from build123d import *

# Parameters (mm, degrees)
ESQUISSE1_R         = 20
ESQUISSE1_R_2       = 12.7
BOSS_EXTRU_1_DEPTH  = 8.78
ESQUISSE2_R         = 38
ESQUISSE2_R_2       = 11.2
BOSS_EXTRU_2_DEPTH  = 47.8
CHANFREIN3_SIZE     = 11.200084029
CHANFREIN3_SIZE_2   = 49.8
SKETCH7_R           = 38
SKETCH7_R_2         = 26
CUT_EXTRUDE2_DEPTH  = 3
CIRPATTERN1_COUNT   = 3
CIRPATTERN2_COUNT   = 3
SKETCH23_R          = 13.7
SKETCH23_R_2        = 12.6
BOSS_EXTRUDE1_DEPTH = 0.3
LPATTERN1_COUNT     = 8
LPATTERN1_PITCH     = 5


with BuildPart() as part:
    # Esquisse1 → Boss.-Extru.1 (new body)
    with BuildSketch(Plane.XY):
        Circle(ESQUISSE1_R)
        Circle(ESQUISSE1_R_2, mode=Mode.SUBTRACT)
    extrude(amount=BOSS_EXTRU_1_DEPTH)

    # Esquisse2 → Boss.-Extru.2 (add)
    with BuildSketch(Plane(origin=(0, 0, 0), x_dir=(-1, 0, 0), z_dir=(0, 0, -1))):
        with Locations(Location((0, 0, 0), (0, 0, 180))):
            Circle(ESQUISSE2_R)
        with Locations(Location((0, 0, 0), (0, 0, 180))):
            Circle(ESQUISSE2_R_2, mode=Mode.SUBTRACT)
    extrude(amount=BOSS_EXTRU_2_DEPTH)

    # Chanfrein3
    # the kernel refuses this chamfer: 49.8, 11.200084029 mm, written as the material it takes off along each edge
    with BuildSketch(Plane(origin=(0, 0, -47.8), x_dir=(1, 0, 0), z_dir=(0, 1, 0))) as chanfrein3_piece_1:
        Polygon((11.2 + CHANFREIN3_SIZE, 0), (11.2, -CHANFREIN3_SIZE_2), (11.2, 0), align=None)
    revolve(axis=Axis((0, 0, -47.8), (0, 0, -1)), mode=Mode.SUBTRACT)

    # Sketch7 → Cut-Extrude2 (cut)
    with BuildSketch(Plane.XY):
        Circle(SKETCH7_R)
        Circle(SKETCH7_R_2, mode=Mode.SUBTRACT)
    cut_extrude2 = extrude(amount=-CUT_EXTRUDE2_DEPTH, mode=Mode.SUBTRACT)

    # Sketch19 → Hole for #4 300® SC Nuts (SP)2 (revolve, cut)
    with BuildSketch(Plane(origin=(28.837585054, 8.270047658, -47.8), x_dir=(0, 1, 0), z_dir=(1, 0, 0))):
        Polygon((0, 0), (0, 6.266734357), (2.1082, 5), (2.1082, 0), align=None)
    hole_for_4_300_sc_nuts_sp_2 = revolve(axis=Axis((28.837585054, 8.270047658, -54.15), (0, 0, 1)), mode=Mode.SUBTRACT)

    # CirPattern1: Hole for #4 300® SC Nuts (SP)2 ×3 about axis
    cirpattern1_axis = Axis((0, 0, 0), (0, 0, 1))
    for i in range(1, CIRPATTERN1_COUNT):
        add(hole_for_4_300_sc_nuts_sp_2.rotate(cirpattern1_axis, i * 360 / CIRPATTERN1_COUNT), mode=Mode.SUBTRACT)

    # Sketch22 → Hole for #4 300® SC Nuts (SP)3 (revolve, cut)
    with BuildSketch(Plane(origin=(15.86067178, 4.548526212, 8.78), x_dir=(0, -1, 0), z_dir=(1, 0, 0))):
        Polygon((0, 0), (0, 6.266734357), (2.1082, 5), (2.1082, 0), align=None)
    hole_for_4_300_sc_nuts_sp_3 = revolve(axis=Axis((15.86067178, 4.548526212, 15.13), (0, 0, -1)), mode=Mode.SUBTRACT)

    # CirPattern2: Hole for #4 300® SC Nuts (SP)3 ×3 about axis
    cirpattern2_axis = Axis((0, 0, 0), (0, 0, 1))
    for i in range(1, CIRPATTERN2_COUNT):
        add(hole_for_4_300_sc_nuts_sp_3.rotate(cirpattern2_axis, i * 360 / CIRPATTERN2_COUNT), mode=Mode.SUBTRACT)

    # Sketch23 → Boss-Extrude1 (add)
    with BuildSketch(Plane.XY):
        Circle(SKETCH23_R)
        Circle(SKETCH23_R_2, mode=Mode.SUBTRACT)
    extrude(amount=BOSS_EXTRUDE1_DEPTH)

    # LPattern1: Cut-Extrude2 ×8
    with Locations(*[(0, 0, -i * LPATTERN1_PITCH) for i in range(1, LPATTERN1_COUNT)]):
        add(cut_extrude2, mode=Mode.SUBTRACT)


solid = part.part
Input: part model. Units: mm. Frame: model coordinates. A direction names the side the tool comes from. Coordinates: 2 decimals unless noted, no trailing zeros. Loops run counter-clockwise (first coordinate to the right, second up) from the corner with the lowest first, then second, coordinate; pieces in that order, holes last. Notation, with made-up numbers: (-12, 54.5) - (39, 54.5) arc R19 cw to (39, 83.5) - close; hole circle Ø10 at (-29.75, -20). An arc over 180 degrees is marked (long way). Answer in a Markdown table with one row per item. Add a question column.
Item 1: Access query for faces 1 (the cylindrical face through (-20.633, -15.821, -21.479)), 2 (the flat face through (9.3, 7.4, 0)), 3 (the cylindrical face through (-8.238, 37.096, -28.986)). Directions: +Z, -Z, +X, -X, +Y, -Y. A direction counts if a zero-diameter tool reaches every point of the face in a straight line with its end or side. Return the directions, or none.
Item 2: Section query C-C on z = -4. Return the cut outline in (x, y), then the cut area to 3 significant figures.
Item 3: Line query: line 1 along X through (y, z) = (8.5, -42); line 2 along Z through (x, y) = (18, -14); line 3 along Y through (x, z) = (2, -43). Output: solid intervals per line, ascending. Write a range as [from, to].
Item 4: Section query B-B on z = -40. Return the cut outline in (x, y), then the cut area to 3 significant figures.
Item 5: Section query A-A on x = -32. State how many separate pieces and enclosed holes the cut face has, then the cut area to 3 significant figures.
Item 6: Contact query for flat-ended pins moving along their axis: P1, Ø10, axis at x = 18.5, z = -24.5, coming from the -Y side; P2, Ø6, axis at x = -29, z = -37.5, coming from the -Y side; P3, Ø12.5, axis at x = 2.5, y = 4.5, coming from the +Z side; P4, Ø3.5, axis at x = 15.86, y = 4.55, coming from the +Z side. Output: stop coordinate, or through.
Item 7: Mould query, pull axis X, two halves, no side actions, for faces 4 (the flat face through (25, -8, -25)), 5 (the cylindrical face through (-8.238, 37.096, -3.986)), 6 (the cylindrical face through (-22.21, 22.85, -45.33)). Classes: released by +X, released by -X, zero draft, split by the parting line, or undercut.
Recorded:
| question | item | result |
|---|---|---|
| 1 | face 1 | none |
| 1 | face 2 | +Z |
| 1 | face 3 | +Z, -Z |
| 2 | outline | circle Ø76 at (0, 0); hole circle Ø25.1 at (0, 0) |
| 2 | area | 4,040 mm^2 |
| 3 | line 1 | [-37.04, -19.31], [19.31, 28.1], [29.58, 37.04] |
| 3 | line 2 | [-47.8, 0] |
| 3 | line 3 | [-37.95, -21.23], [21.23, 37.95] |
| 4 | outline | circle Ø76 at (0, 0); hole circle Ø41.29 at (0, 0) |
| 4 | area | 3,200 mm^2 |
| 5 | separate pieces | 8 |
| 5 | enclosed holes | 0 |
| 5 | area | 976 mm^2 |
| 6 | P1 | y = -35.52 |
| 6 | P2 | y = -27.67 |
| 6 | P3 | through |
| 6 | P4 | z = 3.57 |
| 7 | face 4 | zero draft |
| 7 | face 5 | split by the parting line |
| 7 | face 6 | undercut |
